```python
from build123d import *

# Parameters (mm, degrees)
SKETCH1_R           = 11
SKETCH1_R_2         = 6.4
BOSS_EXTRUDE1_DEPTH = 10
SKETCH1_3_R         = 6.4
BOSS_EXTRUDE2_DEPTH = 24


with BuildPart() as part:
    # Sketch1 → Boss-Extrude1 (new body, symmetric)
    with BuildSketch(Plane.XY):
        Circle(SKETCH1_R)
        Circle(SKETCH1_R_2, mode=Mode.SUBTRACT)
    extrude(amount=BOSS_EXTRUDE1_DEPTH, both=True)

    # Sketch1_3 → Boss-Extrude2 (add, symmetric)
    with BuildSketch(Plane.XY):
        Polygon((-9.526279442, 5.5), (-9.526279442, -5.5), (0, -11), (9.526279442, -5.5), (9.526279442, 5.5), (0, 11), align=None)
        Circle(SKETCH1_3_R, mode=Mode.SUBTRACT)
    extrude(amount=BOSS_EXTRUDE2_DEPTH, both=True)


solid = part.part
```
Work out the finished part from the listing and answer in its coordinate system (mm). A direction names the side the tool comes from. Coordinates: 2 decimals unless noted, no trailing zeros. Order: outer loops, then holes, each group sorted by start corner. A loop starts at its lowest first (then second) coordinate and runs counter-clockwise, first axis right, second up. Notation, with made-up numbers: M 74,12 L 109,12 A7 ccw 109,22 Z; hole C -7.5,21 d7. An arc over 180 degrees is marked long. Use CSV: the item, a comma, the result in double quotes.
1) Flat-ended cylindrical pins translate along their axes: pin 1 Ø1.7 at (x, y) = (-6.5, -8.5) entering from -Z; pin 2 Ø4 at (x, z) = (2, -0.5) entering from -Y; pin 3 Ø5 at (x, z) = (-8.5, -16) entering from +Y; pin 4 Ø2 at (y, z) = (-2, -3) entering from -X. Find the tip coordinate at first contact, or state that the pin passes through.
Worked out:
pin 1,"stops at z = -10"
pin 2,"stops at y = -11"
pin 3,"stops at y = 7.54"
pin 4,"stops at x = -10.95"
2) Section A-A on z = 20.5 is taken. Write down the section's boundary in (x, y), plus the area to 3 significant figures.
Worked out:
outline,"M -9.53,-5.5 L 0,-11 L 9.53,-5.5 L 9.53,5.5 L 0,11 L -9.53,5.5 Z; hole C 0,0 d12.8"
area,"186 mm^2"
3) Section D-D on y = 7 is taken. Write down the section's boundary in (x, z).
Worked out:
outline,"M -8.49,-10 L -6.93,-10 L -6.93,-24 L 6.93,-24 L 6.93,-10 L 8.49,-10 L 8.49,10 L 6.93,10 L 6.93,24 L -6.93,24 L -6.93,10 L -8.49,10 Z"
4) Consider line 1 (Y direction, x = 0, z = 13); line 2 (Z direction, x = 4.5, y = -10); line 3 (Y direction, x = -5.25, z = -18.5). Determine where each line is inside the solid, lowest interval first. Write a range as [from, to].
Worked out:
line 1,"y = [-11, -6.4], [6.4, 11]"
line 2,"z = [-10, 10]"
line 3,"y = [-7.97, -3.66], [3.66, 7.97]"
5) Section C-C on x = 5.75 is taken. Write down the section's boundary in (y, z), plus the area to 3 significant figures.
Worked out:
outline,"M -9.38,-10 L -7.68,-10 L -7.68,-24 L -2.81,-24 L -2.81,24 L -7.68,24 L -7.68,10 L -9.38,10 Z; M 2.81,-24 L 7.68,-24 L 7.68,-10 L 9.38,-10 L 9.38,10 L 7.68,10 L 7.68,24 L 2.81,24 Z"
area,"535 mm^2"
6) Section B-B on y = -1.5 is taken. Write down the section's boundary in (x, z).
Worked out:
outline,"M -10.9,-10 L -9.53,-10 L -9.53,-24 L -6.22,-24 L -6.22,24 L -9.53,24 L -9.53,10 L -10.9,10 Z; M 6.22,-24 L 9.53,-24 L 9.53,-10 L 10.9,-10 L 10.9,10 L 9.53,10 L 9.53,24 L 6.22,24 Z"
7) For faces 1 (the face through (-5, 9, 10)), 2 (the face through (-5, -9, -10)), 3 (the face through (5, -9, 10)), determine the directions among +Z, -Z, +X, -X, +Y, -Y from which every point of the face is accessible in a straight line to the end or side of a thin tool.
Worked out:
face 1,"+Z, -X, +Y"
face 2,"-Z, -X, -Y"
face 3,"+Z, +X, -Y"
